from build123d import *

# Parameters (mm, degrees)
F0_R      = 11
F1_DEPTH  = 67
F3_R      = 11
F3_R_2    = 9.5
F4_DEPTH  = 70
F6_R      = 11
F6_R_2    = 8
F7_DEPTH  = 39.001
F8_R      = 4.15
F9_DEPTH  = 44
F11_R     = 4.15
F12_DEPTH = 20.501


with BuildPart() as f1:
    # F0 (on Right) → F1 (new body, symmetric)
    with BuildSketch(Plane.YZ):
        Circle(F0_R)
    extrude(amount=F1_DEPTH, both=True)

    # F3 (on offset) → F4 (cut)
    with BuildSketch(Plane.YZ.offset(42)):
        Circle(F3_R)
        Circle(F3_R_2, mode=Mode.SUBTRACT)
    extrude(amount=-F4_DEPTH, mode=Mode.SUBTRACT)

    # F6 (on offset) → F7 (cut, through all)
    with BuildSketch(Plane.YZ.offset(-28)):
        Circle(F6_R)
        Circle(F6_R_2, mode=Mode.SUBTRACT)
    extrude(amount=-F7_DEPTH, mode=Mode.SUBTRACT)

    # F8 (on face) → F9 (cut)
    with BuildSketch(Plane.YZ.offset(67)):
        Circle(F8_R)
    extrude(amount=-F9_DEPTH, mode=Mode.SUBTRACT)

    # F11 (on offset) → F12 (cut, through all)
    with BuildSketch(Plane.XY.offset(9.5)):
        with Locations((30, 0)):
            Circle(F11_R)
    extrude(amount=-F12_DEPTH, mode=Mode.SUBTRACT)


solid = f1.part
Part model, mm, in its own coordinate system. A direction names the side the tool comes from. Coordinates: 2 decimals unless noted, no trailing zeros. Order: outer loops, then holes, each group sorted by start corner. A loop starts at its lowest first (then second) coordinate and runs counter-clockwise, first axis right, second up.
(1) Pull direction X, two halves, no side cores. Call faces 4 (the face through (-28, -4.3, -7)), 5 (the face through (25.854, 0.182, -5.743)), 6 (the face through (-47.23, -1.73, -7.81)): pulls with the +X half, pulls with the -X half, needs draft (parallel to the pull), parting line crosses it, or undercut.
Check sheet entries:
face 4: pulls with the -X half
face 5: undercut
face 6: needs draft
(2) Slice it at A-A, the plane y = 0. Write the cut outline in (x, z), and give its area (3 significant figures).
Check sheet entries:
outline: (-67, -8) - (-28, -8) - (-28, -9.5) - (25.85, -9.5) - (25.85, -4.15) - (23, -4.15) - (23, 4.15) - (25.85, 4.15) - (25.85, 9.5) - (-28, 9.5) - (-28, 8) - (-67, 8) - close; (34.15, -9.5) - (42, -9.5) - (42, -11) - (67, -11) - (67, -4.15) - (34.15, -4.15) - close; (34.15, 4.15) - (67, 4.15) - (67, 11) - (42, 11) - (42, 9.5) - (34.15, 9.5) - close
area: 2,050 mm2
(3) Tool access for faces 1 (the face through (54.68, -2.38, -10.74)), 2 (the face through (23, 0, 0)), 3 (the face through (42, -10, 0)): list every direction of +Z, -Z, +X, -X, +Y, -Y with a clear straight run to the whole face (end or side of a thin tool).
Check sheet entries:
face 1: +X, -X
face 2: +X
face 3: -X
(4) Slice it at B-B, the plane x = 38.5. Write the cut outline in (y, z).
Check sheet entries:
outline: circle Ø19 at (0, 0); hole circle Ø8.3 at (0, 0)
(5) Pin check, flat tips, straight feed: pin 1 Ø1 at (y, z) = (-1.5, -2) entering from +X; pin 2 Ø3 at (y, z) = (-7.5, -7) entering from -X; pin 3 Ø1 at (x, z) = (0, 6.5) entering from +Y; pin 4 Ø5 at (y, z) = (2, 8.5) entering from -X. Stop position of each tip, or through.
Check sheet entries:
pin 1: stops at x = 23
pin 2: stops at x = -28
pin 3: stops at y = 7.37
pin 4: stops at x = -67
(6) Probe L1, parallel to Y at x = 36.5, z = 0.25; L2, parallel to X at y = 0, z = -6; L3, parallel to Z at x = 36, y = 0. List the from-to ranges inside material, lowest first.
Check sheet entries:
L1: y = -9.5 to -4.14, 4.14 to 9.5
L2: x = -67 to 25.85, 34.15 to 67
L3: z = -9.5 to -4.15, 4.15 to 9.5
(7) Slice it at D-D, the plane x = -43. Write the cut outline in (y, z).
Check sheet entries:
outline: circle Ø16 at (0, 0)
(8) Slice it at C-C, the plane z = -5.5. Write the cut outline in (x, y).
Check sheet entries:
outline: (-67, -5.81) - (-28, -5.81) - (-28, -7.75) - (42, -7.75) - (42, -9.53) - (67, -9.53) - (67, 9.53) - (42, 9.53) - (42, 7.75) - (-28, 7.75) - (-28, 5.81) - (-67, 5.81) - close; hole circle Ø8.3 at (30, 0)
